Geometry check sheet. Reference: the model listing, model coordinates, mm. Give positions to 0.01 mm unless a question says otherwise; leave off trailing zeros. Loops run counter-clockwise (first coordinate to the right, second up) from the corner with the lowest first, then second, coordinate; pieces in that order, holes last. Notation, with made-up numbers: (33, -14.5) -> (58, -14.5) arc R20 ccw to (58, 14.5) -> close; hole circle Ø1 at (-3, 71). An arc over 180 degrees is marked (long way). One line per question, with ' | ' between items.
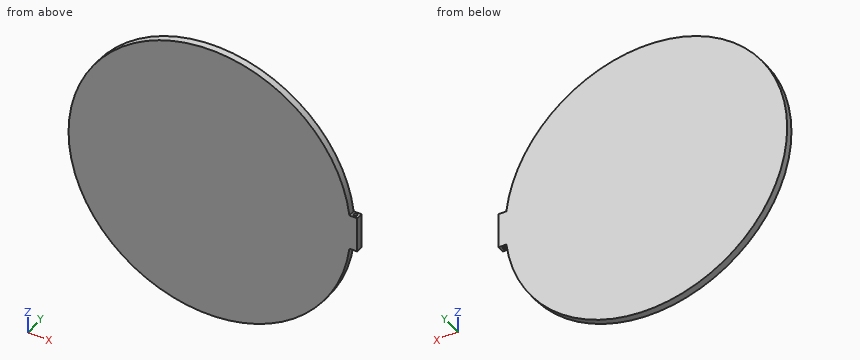
from build123d import *

# Parameters (mm, degrees)
BOSS_EXTRUDE1_DEPTH = 2.54
SKETCH2_R           = 0.635
CUT_EXTRUDE1_DEPTH  = 119.691411293


with BuildPart() as part:
    # Sketch1 → Boss-Extrude1 (new body)
    with BuildSketch(Plane(origin=(0, 0, 0), x_dir=(1, 0, 0), z_dir=(0, 1, 0))):
        with BuildLine():
            Line((0, 0), (0, 12.7))
            Line((0, 12.7), (-2.794, 12.7))
            ThreePointArc((-2.794, 12.7), (-103.995562476, 6.35), (-2.794, 0))
            Line((-2.794, 0), (0, 0))
        make_face()
    extrude(amount=BOSS_EXTRUDE1_DEPTH)

    # Sketch2 → Cut-Extrude1 (cut, through all)
    with BuildSketch(Plane.XY):
        with Locations((-1.397, 1.27)):
            Circle(SKETCH2_R)
    extrude(amount=-CUT_EXTRUDE1_DEPTH, mode=Mode.SUBTRACT)


solid = part.part
Item 1: Scan lines: probe 1 along X at (y, z) = (2.15, -7.5); probe 2 along Z at (x, y) = (-7.5, 0.8); probe 3 along Z at (x, y) = (-71, 2.4). Record each from-to range of solid material in increasing order.
Result:
probe 1: -103.98 to 0 | probe 2: -28.54 to 15.84 | probe 3: -53.93 to 41.23
Item 2: Depth check by flat-ended pin: pin 1 Ø1.5 at (y, z) = (2, -21) entering from +X; pin 2 Ø2 at (x, z) = (-14.5, 29) entering from +Y; pin 3 Ø0.8 at (x, y) = (-2, 1) entering from -Z. Enter the tip coordinate at first touch or a pass-through.
Result:
pin 1: x = -4.33 | pin 2: through | pin 3: z = -12.7
Item 3: Sectioned sample at A-A (y = 1.27). Record the cut outline in (x, z), plus the area to 3 significant figures.
Result:
outline: (-2.79, -12.7) -> (-2.03, -12.7) -> (-2.03, 0) -> (-2.79, 0) arc R50.8 ccw (long way) to start; (-0.76, -12.7) -> (0, -12.7) -> (0, 0) -> (-0.76, 0) -> close | area: 8,120 mm2
Item 4: Sectioned sample at B-B (z = 2). Record the cut outline in (x, y), plus the area to 3 significant figures.
Result:
outline: (-103.3, 0) -> (-3.09, 0) -> (-3.09, 2.54) -> (-103.3, 2.54) -> close | area: 255 mm2
Item 5: Sectioned sample at C-C (x = -72). Record the cut outline in (y, z), plus the area to 3 significant figures.
Result:
outline: (0, -53.54) -> (2.54, -53.54) -> (2.54, 40.84) -> (0, 40.84) -> close | area: 240 mm2
